Check sheet for the drawn part. Datum: minimum x, y, z corner. Units: mm. A direction names the side the tool comes from. Round coordinates to 2 decimals unless told otherwise and drop trailing zeros. Write each loop counter-clockwise with the first axis right and the second up, starting at its lowest first coordinate (ties: lowest second). Pieces come first, ordered by that corner, then holes. Notation, with made-up numbers: M 77,4.25 L 132,4.25 A27 cw 132,37.25 Z; hole C 56,-5.75 d5. An arc over 180 degrees is marked long. One line per item, written item: value.
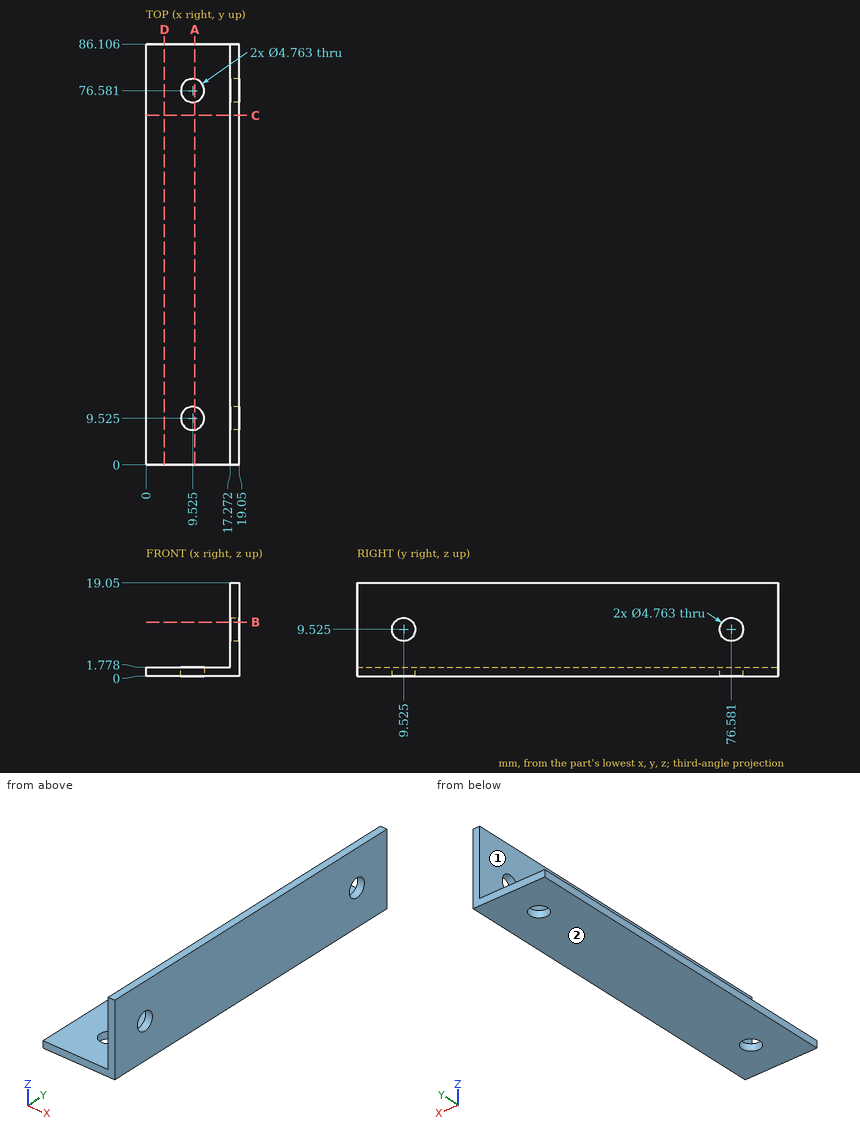
Q1. Depth check by flat-ended pin: P1, Ø5, axis at y = 65.5, z = 16.5, coming from the -X side; P2, Ø8.5, axis at x = 9, y = 43, coming from the +Z side. Enter the tip coordinate at first touch or a pass-through.
Completed:
P1: x = 17.27
P2: z = 1.78
Q2. Sectioned sample at B-B on z = 11. State how many separate pieces and enclosed holes the cut face has, and give its area (3 significant figures).
Completed:
separate pieces: 3
enclosed holes: 0
area: 140 mm^2
Q3. Sectioned sample at D-D on x = 3.75. Enter the section's corners in (y, z) (1 decimal), and give its area (3 significant figures).
Completed:
outline: M 0,0 L 86.1,0 L 86.1,1.8 L 0,1.8 Z
area: 153 mm^2
Q4. Scan lines: line 1 (Z direction, x = 14.25, y = 34); line 2 (X direction, y = 61, z = 17.5). Record each from-to range of solid material in increasing order. Write a range as [from, to].
Completed:
line 1: [0, 1.78]
line 2: [17.27, 19.05]
Q5. Access from +Z, -Z, +X, -X, +Y, -Y to the whole of each face (thin tool, end or side, straight path). Record for the marked faces 1 and 2.
Completed:
face 1: +Z, -X, +Y, -Y
face 2: -Z, +X, -X, +Y, -Y
Q6. Sectioned sample at A-A on x = 10. Enter the section's corners in (y, z) (1 decimal).
Completed:
outline: M 0,0 L 7.2,0 L 7.2,1.8 L 0,1.8 Z; M 11.9,0 L 74.2,0 L 74.2,1.8 L 11.9,1.8 Z; M 78.9,0 L 86.1,0 L 86.1,1.8 L 78.9,1.8 Z
Q7. Sectioned sample at C-C on y = 71.5. Enter the section's corners in (x, z).
Completed:
outline: M 0,0 L 19.05,0 L 19.05,19.05 L 17.27,19.05 L 17.27,1.78 L 0,1.78 Z
